Could you check a few things on this model? Use its own coordinates, in mm. A direction names the side the tool comes from. Round coordinates to 2 decimals unless told otherwise and drop trailing zeros. Loops run counter-clockwise (first coordinate to the right, second up) from the corner with the lowest first, then second, coordinate; pieces in that order, holes last. Notation, with made-up numbers: (45, -18.5) -> (85, -18.5) arc R19 cw to (85, 15.5) -> close; hole circle Ø9 at (87, -38). An arc over 180 degrees is marked (long way). One line per item, written item: value.
from build123d import *

# Parameters (mm, degrees)
SKETCH1_W           = 15
SKETCH1_H           = 14
BOSS_EXTRUDE1_DEPTH = 10
SKETCH2_R           = 1.8
CUT_EXTRUDE1_DEPTH  = 17.26246018
SKETCH3_R           = 2
CUT_EXTRUDE2_DEPTH  = 5
SKETCH4_W           = 3.5
SKETCH4_H           = 10
BOSS_EXTRUDE2_DEPTH = 8
SKETCH5_W           = 15
SKETCH5_H           = 10
BOSS_EXTRUDE3_DEPTH = 4
SKETCH6_R           = 1.65
CUT_EXTRUDE3_DEPTH  = 4


with BuildPart() as part:
    # Sketch1 → Boss-Extrude1 (new body)
    with BuildSketch(Plane.XY):
        with Locations((-0.595285601, 2.94655529)):
            Rectangle(SKETCH1_W, SKETCH1_H)
    extrude(amount=BOSS_EXTRUDE1_DEPTH)

    # Sketch2 → Cut-Extrude1 (cut, through all)
    with BuildSketch(Plane.XY.offset(10)):
        with Locations((-0.595285601, 2.94655529)):
            Circle(SKETCH2_R)
    extrude(amount=-CUT_EXTRUDE1_DEPTH, mode=Mode.SUBTRACT)

    # Sketch3 → Cut-Extrude2 (cut)
    with BuildSketch(Plane(origin=(0, 9.94655529, 0), x_dir=(1, 0, 0), z_dir=(0, 1, 0))):
        with Locations(Location((-0.595285601, -5, 0), (0, 0, 270))):
            Circle(SKETCH3_R)
    extrude(amount=-CUT_EXTRUDE2_DEPTH, mode=Mode.SUBTRACT)

    # Sketch4 → Boss-Extrude2 (add)
    with BuildSketch(Plane(origin=(0, 9.94655529, 0), x_dir=(1, 0, 0), z_dir=(0, 1, 0))):
        with Locations((-6.345285601, -5)):
            Rectangle(SKETCH4_W, SKETCH4_H)
        with Locations((5.154714399, -5)):
            Rectangle(SKETCH4_W, SKETCH4_H)
    extrude(amount=BOSS_EXTRUDE2_DEPTH)

    # Sketch5 → Boss-Extrude3 (add)
    with BuildSketch(Plane(origin=(0, 17.94655529, 0), x_dir=(1, 0, 0), z_dir=(0, 1, 0))):
        with Locations((-0.595285601, -5)):
            Rectangle(SKETCH5_W, SKETCH5_H)
    extrude(amount=BOSS_EXTRUDE3_DEPTH)

    # Sketch6 → Cut-Extrude3 (cut)
    with BuildSketch(Plane(origin=(0, 21.94655529, 0), x_dir=(1, 0, 0), z_dir=(0, 1, 0))):
        with Locations(Location((-0.595285601, -5, 0), (0, 0, 270))):
            Circle(SKETCH6_R)
    extrude(amount=-CUT_EXTRUDE3_DEPTH, mode=Mode.SUBTRACT)


solid = part.part
(1) If we section it at D-D, the plane z = 1.25: Please give me the cut outline in (x, y).
Recorded:
outline: (-8.1, -4.05) -> (6.9, -4.05) -> (6.9, 21.95) -> (-8.1, 21.95) -> close; hole (-4.6, 9.95) -> (3.4, 9.95) -> (3.4, 17.95) -> (-4.6, 17.95) -> close; hole circle Ø3.6 at (-0.6, 2.95)
(2) If I drill on L1, parallel to Y at x = -0.5, z = 8.25; L2, parallel to Y at x = 1.5, z = 7.25; L3, parallel to X at y = 18.9, z = 5, over which ranges is the centre line in solid material (lowest first)?
Recorded:
L1: -4.05 to 1.15, 4.74 to 9.95, 17.95 to 21.95
L2: -4.05 to 9.95, 17.95 to 21.95
L3: -8.1 to -2.25, 1.05 to 6.9
(3) If we section it at A-A, the plane x = 2.5: Please give me the cut outline in (y, z).
Recorded:
outline: (-4.05, 0) -> (9.95, 0) -> (9.95, 10) -> (-4.05, 10) -> close; (17.95, 0) -> (21.95, 0) -> (21.95, 10) -> (17.95, 10) -> close
(4) If we section it at B-B, the plane y = 17: Please give me the cut outline in (x, z).
Recorded:
outline: (-8.1, 0) -> (-4.6, 0) -> (-4.6, 10) -> (-8.1, 10) -> close; (3.4, 0) -> (6.9, 0) -> (6.9, 10) -> (3.4, 10) -> close
(5) Thinking about a two-plate mould opening in Z: for faces 4 (the face through (-2.4, 21.947, 4.9)), 5 (the face through (-0.52, 19.97, 3.35)), 6 (the face through (-0.51, 7.48, 3)), 7 (the face through (-1, 9, 10)), which applies, released by +Z, released by -Z, zero draft, split by the parting line, or undercut?
Recorded:
face 4: zero draft
face 5: undercut
face 6: undercut
face 7: released by +Z
(6) For faces 1 (the face through (-1, -4.053, 5)), 2 (the face through (-2.4, 17.947, 4.9)), 3 (the face through (-1, 4.947, 5)), which set-ups out of +Z, -Z, +X, -X, +Y, -Y let a thin tool reach every point of the face, with its end or its side?
Recorded:
face 1: +Z, -Z, +X, -X, -Y
face 2: +Z, -Z
face 3: none
(7) If we section it at C-C, the plane z = 4.5: Please give me the cut outline in (x, y).
Recorded:
outline: (-8.1, -4.05) -> (6.9, -4.05) -> (6.9, 21.95) -> (0.98, 21.95) -> (0.98, 17.95) -> (3.4, 17.95) -> (3.4, 9.95) -> (1.34, 9.95) -> (1.34, 4.95) -> (-2.53, 4.95) -> (-2.53, 9.95) -> (-4.6, 9.95) -> (-4.6, 17.95) -> (-2.17, 17.95) -> (-2.17, 21.95) -> (-8.1, 21.95) -> close; hole circle Ø3.6 at (-0.6, 2.95)
